from build123d import *

# Parameters (mm, degrees)
SKETCH1_W           = 24.9
SKETCH1_H           = 16
SKETCH1_W_2         = 18.9
SKETCH1_H_2         = 10
BOSS_EXTRUDE1_DEPTH = 1
SKETCH2_W           = 24.9
SKETCH2_H           = 16
SKETCH2_W_2         = 20.9
SKETCH2_H_2         = 12
BOSS_EXTRUDE2_DEPTH = 8
SKETCH3_W           = 2
SKETCH3_H           = 16
BOSS_EXTRUDE3_DEPTH = 15
FILLET1_R           = 5
SKETCH4_R           = 1.4
CUT_EXTRUDE1_DEPTH  = 24.9
FILLET2_R           = 6


with BuildPart() as part:
    # Sketch1 → Boss-Extrude1 (new body)
    with BuildSketch(Plane(origin=(0, 0, 0), x_dir=(1, 0, 0), z_dir=(0, 1, 0))):
        Rectangle(SKETCH1_W, SKETCH1_H)
        Rectangle(SKETCH1_W_2, SKETCH1_H_2, mode=Mode.SUBTRACT)
    extrude(amount=BOSS_EXTRUDE1_DEPTH)

    # Sketch2 → Boss-Extrude2 (add)
    with BuildSketch(Plane(origin=(0, 1, 0), x_dir=(1, 0, 0), z_dir=(0, 1, 0))):
        Rectangle(SKETCH2_W, SKETCH2_H)
        Rectangle(SKETCH2_W_2, SKETCH2_H_2, mode=Mode.SUBTRACT)
    extrude(amount=BOSS_EXTRUDE2_DEPTH)

    # Sketch3 → Boss-Extrude3 (add)
    with BuildSketch(Plane(origin=(0, 9, 0), x_dir=(1, 0, 0), z_dir=(0, 1, 0))):
        with Locations((-11.45, 0)):
            Rectangle(SKETCH3_W, SKETCH3_H)
        with Locations((11.45, 0)):
            Rectangle(SKETCH3_W, SKETCH3_H)
    extrude(amount=BOSS_EXTRUDE3_DEPTH)

    # Fillet1
    fillet1_edges = [part.edges().sort_by_distance(p)[0] for p in [
        (-10.45, 9, -7),
        (-10.45, 9, 7),
        (10.45, 9, 7),
        (10.45, 9, -7),
    ]]
    fillet(fillet1_edges, radius=FILLET1_R)

    # Sketch4 → Cut-Extrude1 (cut)
    with BuildSketch(Plane(origin=(12.45, 0, 0), x_dir=(0, 0, -1), z_dir=(1, 0, 0))):
        with Locations((0, 21.1)):
            Circle(SKETCH4_R)
    extrude(amount=-CUT_EXTRUDE1_DEPTH, mode=Mode.SUBTRACT)

    # Fillet2
    fillet2_edges = [part.edges().sort_by_distance(p)[0] for p in [
        (11.45, 24, -8),
        (11.45, 24, 8),
        (-11.45, 24, 8),
        (-11.45, 24, -8),
    ]]
    fillet(fillet2_edges, radius=FILLET2_R)


solid = part.part
For this review, take the finished solid that the model builds, in its own axes (mm). A direction names the side the tool comes from. Round coordinates to 2 decimals unless told otherwise and drop trailing zeros. Order: outer loops, then holes, each group sorted by start corner. A loop starts at its lowest first (then second) coordinate and runs counter-clockwise, first axis right, second up. Notation, with made-up numbers: M 46,-7 L 61,-7 A25 cw 61,31 Z; hole C -16,4.25 d6. An arc over 180 degrees is marked long. Use a Markdown table: item, result. Add a question column.
Item 1: Mouldability with a two-part tool opening along X and no side actions: class faces 1 (the cylindrical face through (-11.436, 22.196, 6.289)), 2 (the flat face through (-0.1, 0.5, -5)) as released by +X, released by -X, zero draft, split by the parting line, or undercut.
Item 2: To check wall thickness, follow line 1 along X through (y, z) = (21, 2.75); line 2 along Y through (x, z) = (-10.9, 0); line 3 along Z through (x, y) = (6, 2). State the ranges of each line that lie inside material, in increasing order.
Item 3: Insertion check: pin 1 (1 mm diameter, centred on x = -1.5, z = -6.5, fed in from +Y). The pin has a flat end and moves straight along its axis. Give the tip position at first contact, or say it passes through.
Item 4: Add section D-D, the plane y = 19. Give the boundary of the cut face in (x, z).
Item 5: Add section C-C, the plane y = 7.75. Give the boundary of the cut face in (x, z).
Item 6: Tool access review of faces 3 (the flat face through (9.45, 0.5, 0.1)), 4 (the flat face through (0, 9, 7)), 5 (the cylindrical face through (11.46, 22.28, -0.75)), 6 (the flat face through (0, 6, 6)): name each direction out of +Z, -Z, +X, -X, +Y, -Y from which nothing blocks a thin tool from reaching the whole face with its end or side.
Item 7: Add section A-A, the plane z = 0. Give the boundary of the cut face in (x, y), then the cut area to 3 significant figures.
Item 8: Add section B-B, the plane x = -2.5. Give the boundary of the cut face in (y, z).
Geometry results:
| question | item | result |
|---|---|---|
| 1 | face 1 | zero draft |
| 1 | face 2 | undercut |
| 2 | line 1 | x = -12.45 to -10.45, 10.45 to 12.45 |
| 2 | line 2 | y = 0 to 19.7, 22.5 to 24 |
| 2 | line 3 | z = -8 to -6, 6 to 8 |
| 3 | pin 1 | stops at y = 9 |
| 4 | outline | M -12.45,-7.92 L -10.45,-7.92 L -10.45,7.92 L -12.45,7.92 Z; M 10.45,-7.92 L 12.45,-7.92 L 12.45,7.92 L 10.45,7.92 Z |
| 5 | outline | M -12.45,-8 L 12.45,-8 L 12.45,8 L -12.45,8 Z; hole M -10.45,-6 L 10.45,-6 L 10.45,6 L -10.45,6 Z |
| 6 | face 3 | +Y, -Y |
| 6 | face 4 | +Z, -Z, +Y |
| 6 | face 5 | +X, -X |
| 6 | face 6 | +Y |
| 7 | outline | M -12.45,0 L -9.45,0 L -9.45,1 L -10.45,1 L -10.45,19.7 L -12.45,19.7 Z; M -12.45,22.5 L -10.45,22.5 L -10.45,24 L -12.45,24 Z; M 9.45,0 L 12.45,0 L 12.45,19.7 L 10.45,19.7 L 10.45,1 L 9.45,1 Z; M 10.45,22.5 L 12.45,22.5 L 12.45,24 L 10.45,24 Z |
| 7 | area | 86.8 mm² |
| 8 | outline | M 0,-8 L 9,-8 L 9,-6 L 1,-6 L 1,-5 L 0,-5 Z; M 0,5 L 1,5 L 1,6 L 9,6 L 9,8 L 0,8 Z |
